Design review of the part built by this model. Coordinates are the model's own, in mm. Face numbers are marked on the shaded views. Round coordinates to 2 decimals unless told otherwise and drop trailing zeros. Loops run counter-clockwise (first coordinate to the right, second up) from the corner with the lowest first, then second, coordinate; pieces in that order, holes last. Notation, with made-up numbers: M 84.5,85 L 103.5,85 A26 ccw 103.5,103 Z; hole C 19,36 d6. An arc over 180 degrees is marked long. Use a Markdown table: item, result.
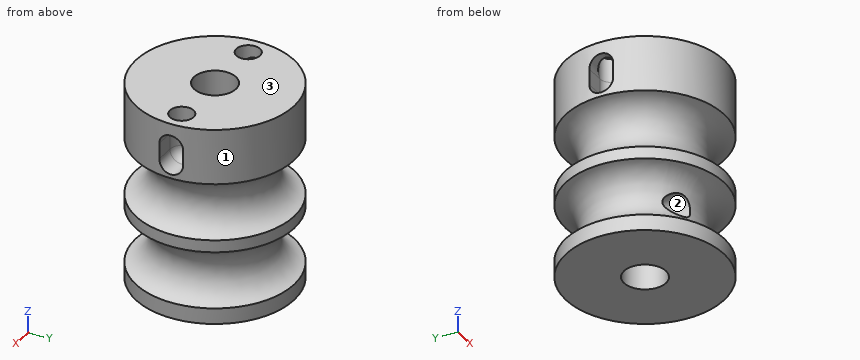
from build123d import *

# Parameters (mm, degrees)
SKETCH029_R      = 1.5
EXTRUDE023_DEPTH = 20
EXTRUDE022_DEPTH = 5
FILLET010_R      = 1.4999
EXTRUDE021_DEPTH = 5
FILLET009_R      = 1.4999
SKETCH026_R      = 1.5
EXTRUDE020_DEPTH = 5


with BuildPart() as extrude023:
    # Sketch029 → Extrude023 (new body)
    with BuildSketch(Plane.XZ):
        with Locations((-3.675, 12.385792)):
            Circle(SKETCH029_R)
    extrude(amount=EXTRUDE023_DEPTH)


with BuildPart() as fillet010:
    # Sketch028 → Extrude022 (new body)
    with BuildSketch(Plane.YZ):
        with BuildLine():
            ThreePointArc((1.5, 27), (0, 28.5), (-1.5, 27))
            Line((-1.5, 27), (-1.5, 25))
            ThreePointArc((-1.5, 25), (0, 23.5), (1.5, 25))
            Line((1.5, 25), (1.5, 27))
        make_face()
    extrude(amount=EXTRUDE022_DEPTH)


with BuildPart() as fillet010_1:
    # Extrude022 placement: moved
    add(fillet010.part.moved(Location((6, 0, 0))))

    # Fillet010
    fillet010_edges = [fillet010_1.edges().sort_by_distance(p)[0] for p in [
        (6, 0, 28.5),
    ]]
    fillet(fillet010_edges, radius=FILLET010_R)


with BuildPart() as fillet010_2:
    # Fillet010 placement: moved
    add(fillet010_1.part.moved(Location((0, 0, 2))))


with BuildPart() as fillet009:
    # Sketch027 → Extrude021 (new body)
    with BuildSketch(Plane.YZ):
        with BuildLine():
            ThreePointArc((1.5, 27), (0, 28.5), (-1.5, 27))
            Line((-1.5, 27), (-1.5, 25))
            ThreePointArc((-1.5, 25), (0, 23.5), (1.5, 25))
            Line((1.5, 25), (1.5, 27))
        make_face()
    extrude(amount=EXTRUDE021_DEPTH)


with BuildPart() as fillet009_1:
    # Extrude021 placement: moved
    add(fillet009.part.moved(Location((6, 0, 0))))

    # Fillet009
    fillet009_edges = [fillet009_1.edges().sort_by_distance(p)[0] for p in [
        (6, 0, 28.5),
    ]]
    fillet(fillet009_edges, radius=FILLET009_R)


with BuildPart() as fillet009_2:
    # Fillet009 placement: moved
    add(fillet009_1.part.moved(Location((0, 0, 2))))


with BuildPart() as fusion008:
    # Part__Mirroring: instance of Fillet009
    add(fillet009_2.part.mirror(Plane(origin=(0, 0, 0), x_dir=(0, -1, 0), z_dir=(1, 0, 0))))

    # Fusion008: union Fillet010
    add(fillet010_2.part)


with BuildPart() as extrude020:
    # Sketch026 → Extrude020 (new body)
    with BuildSketch(Plane.XY):
        with Locations((7.5, 0)):
            Circle(SKETCH026_R)
        with Locations((-7.5, 0)):
            Circle(SKETCH026_R)
    extrude(amount=-EXTRUDE020_DEPTH)


with BuildPart() as extrude020_1:
    # Extrude020 placement: moved
    add(extrude020.part.moved(Location((0, 0, 32))))


with BuildPart() as cut008:
    # Sketch025 → Revolve001 (revolve)
    with BuildSketch(Plane.YZ):
        with BuildLine():
            Line((-2.65, 27), (-2.65, 7))
            Line((-2.65, 7), (-10, 7))
            Line((-10, 7), (-10, 9))
            ThreePointArc((-10, 9), (-7.25, 12.614208), (-10, 16.228416))
            Line((-10, 17.771584), (-10, 16.228416))
            ThreePointArc((-10, 17.771584), (-7.25, 21.385792), (-10, 25))
            Line((-10, 27), (-10, 25))
            Line((-10, 27), (-10, 32))
            Line((-10, 32), (-2.65, 32))
            Line((-2.65, 32), (-2.65, 27))
        make_face()
    revolve(axis=Axis((0, 0, 0), (0, 0, 1)))

    # Cut006: cut Extrude020
    add(extrude020_1.part, mode=Mode.SUBTRACT)

    # Cut007: cut Fusion008
    add(fusion008.part, mode=Mode.SUBTRACT)

    # Cut008: cut Extrude023
    add(extrude023.part, mode=Mode.SUBTRACT)


solid = cut008.part
1. Take a section at B-B on z = 10. Give the boundary of the cut face in (x, y), and give its area (3 significant figures).
Check values:
| item | result |
|---|---|
| outline | C 0,0 d16.62; hole C 0,0 d5.3 |
| area | 195 mm² |
2. The part is to be moulded in two halves that separate along X. For the marked faces 1, 2 and 3, say which applies: pulls with the +X half, pulls with the -X half, needs draft (parallel to the pull), parting line crosses it, or undercut.
Check values:
| item | result |
|---|---|
| face 1 | parting line crosses it |
| face 2 | undercut |
| face 3 | needs draft |
3. Insertion check: pin 1 (2 mm diameter, centred on x = 3, z = 27, fed in from +Y); pin 2 (5 mm diameter, centred on x = 6.5, z = 13, fed in from +Y); pin 3 (2 mm diameter, centred on x = 9, z = 28.5, fed in from -Y); pin 4 (10 mm diameter, centred on x = -3.5, z = 25.5, fed in from +Y). Each pin has a flat end and moves straight along its axis. Give the tip position at first contact, or say it passes through.
Check values:
| item | result |
|---|---|
| pin 1 | stops at y = 9.8 |
| pin 2 | stops at y = 6.38 |
| pin 3 | stops at y = -6 |
| pin 4 | stops at y = 10 |
4. Take a section at C-C on y = -8.25. Count the separate pieces of the cut face and the enclosed holes in it, and give its area (3 significant figures).
Check values:
| item | result |
|---|---|
| separate pieces | 3 |
| enclosed holes | 0 |
| area | 146 mm² |
5. Take a section at A-A on x = 0. Give the boundary of the cut face in (y, z).
Check values:
| item | result |
|---|---|
| outline | M -10,7 L -2.65,7 L -2.65,32 L -10,32 L -10,25 A3.75 cw -10,17.77 L -10,16.23 A3.75 cw -10,9 Z; M 2.65,7 L 10,7 L 10,9 A3.75 cw 10,16.23 L 10,17.77 A3.75 cw 10,25 L 10,32 L 2.65,32 Z |
6. Wall thickness on line 1 along Z through (x, y) = (6.75, -7.25); line 2 along X through (y, z) = (-2, 11.5); line 3 along Y through (x, z) = (7.5, 29.7): over which ranges is each line inside the solid? List them lowest first. Write a range as from..to.
Check values:
| item | result |
|---|---|
| line 1 | z = 7..9.03, 16.2..17.8, 24.97..32 |
| line 2 | x = -7.14..-4.89, -2.46..-1.74, 1.74..7.14 |
| line 3 | y = -6.61..-1.5, 1.5..6.61 |
